Check sheet for the modelled part. Datum: model origin and axes. Units: mm. Face numbers are marked on the shaded views. A direction names the side the tool comes from. Coordinates: 2 decimals unless noted, no trailing zeros. Write each loop counter-clockwise with the first axis right and the second up, starting at its lowest first coordinate (ties: lowest second). Pieces come first, ordered by that corner, then holes. Notation, with made-up numbers: (-29, 24) - (-10, 24) arc R34 cw to (-10, 57) - close; hole circle Ø6 at (-17, 16). An arc over 180 degrees is marked (long way). Use one line per item in the form item = value. Start each with the question number.
1. Cross-section at C-C on y = 11. Record the boundary of the cut face in (x, z).
2. Cross-section at B-B on y = 5.5. Record the boundary of the cut face in (x, z), then the cut area to 3 significant figures.
3. Scan lines: line 1 along X through (y, z) = (1, -0.25); line 2 along Z through (x, y) = (-4, 1.75); line 3 along Y through (x, z) = (-2.25, 2). Record each from-to range of solid material in increasing order.
4. Go/stop test with flat-tipped pins: pin 1 Ø1 at (x, y) = (-2.5, 2.5) entering from +Z; pin 2 Ø1 at (x, z) = (-2, 2.5) entering from +Y; pin 3 Ø3 at (x, z) = (0, -3) entering from +Y. Record where each tip stops, or that it passes through.
5. Tool access check on the marked faces 4 and 5. Record the directions out of +Z, -Z, +X, -X, +Y, -Y that give a thin tool (end or side, any length) a straight path to the whole face; none if there is none.
6. Draft check along Z on the marked faces 1, 2 and 3. Enter one of: +Z half, -Z half, draft (parallel to the pull), parting line (faces both ways), or undercut.
7. Cross-section at A-A on x = -2.75. Record the boundary of the cut face in (y, z).
```python
from build123d import *

# Parameters (mm, degrees)
REVOLVE1_ANGLE          = 45
SKETCH3_W               = 5
SKETCH3_H               = 5
BOSS_EXTRUDE2_DEPTH     = 5
CHAMFER2_SIZE           = 1.5
CUT_EXTRUDE1_DEPTH      = 1
CUT_EXTRUDE1_DEPTH_BACK = 13.35


with BuildPart() as part:
    # Sketch2 → Revolve1 (revolve, symmetric)
    with BuildSketch(Plane.XY) as revolve1_sk:
        Polygon((0, 0), (5, 0), (5, 12.35), (2.5, 12.35), (2.5, 9.85), (0, 7.35), align=None)
    revolve(axis=Axis((-10, 0, 0), (0, 1, 0)), revolution_arc=REVOLVE1_ANGLE / 2)
    revolve(revolve1_sk.sketch, axis=Axis((-10, 0, 0), (0, -1, 0)), revolution_arc=REVOLVE1_ANGLE / 2)

    # Sketch3 → Boss-Extrude2 (add)
    with BuildSketch(Plane(origin=(0, 0, 0), x_dir=(0, 0, -1), z_dir=(1, 0, 0))):
        with Locations((0, 2.5)):
            Rectangle(SKETCH3_W, SKETCH3_H)
    extrude(amount=-BOSS_EXTRUDE2_DEPTH)

    # Chamfer2
    chamfer2_edges = [part.edges().sort_by_distance(p)[0] for p in [
        (-2.658770817, 0, -2.5),
        (-2.658770817, 0, 2.5),
    ]]
    chamfer(chamfer2_edges, length=CHAMFER2_SIZE)

    # Sketch4 → Cut-Extrude1 (cut, two sides)
    with BuildSketch(Plane.XZ) as cut_extrude1_sk:
        with BuildLine():
            Line((-0.761204675, 3.826834324), (4.503631926, 3.826834324))
            ThreePointArc((4.503631926, 3.826834324), (4.213147766, 4.794416604), (3.858192988, 5.740251485))
            Line((3.858192988, 5.740251485), (-0.761204675, 3.826834324))
        make_face()
        with BuildLine():
            Line((-0.761204675, -3.826834324), (4.503631926, -3.826834324))
            ThreePointArc((4.503631926, -3.826834324), (4.213147766, -4.794416604), (3.858192988, -5.740251485))
            Line((3.858192988, -5.740251485), (-0.761204675, -3.826834324))
        make_face()
    extrude(amount=CUT_EXTRUDE1_DEPTH, mode=Mode.SUBTRACT)
    extrude(cut_extrude1_sk.sketch, amount=-CUT_EXTRUDE1_DEPTH_BACK, mode=Mode.SUBTRACT)


solid = part.part
```
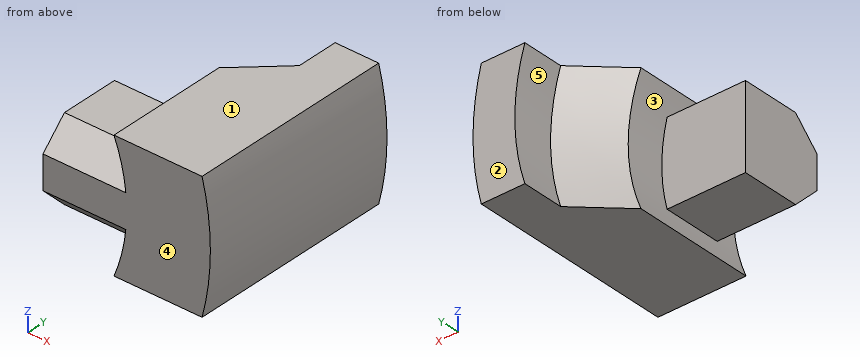
Final values:
q1.outline = (1.9, -3.83) - (4.5, -3.83) arc R15 ccw to (4.5, 3.83) - (1.9, 3.83) arc R12.5 cw to start
q2.outline = (-0.76, -3.83) - (4.5, -3.83) arc R15 ccw to (4.5, 3.83) - (-0.76, 3.83) arc R10 cw to start
q2.area = 38.9 mm²
q3.line_1 = -5 to 5
q3.line_2 = -2.5 to 2.5
q3.line_3 = 1 to 5
q4.pin_1 = 2.5
q4.pin_2 = 5
q4.pin_3 = 9.29
q5.face_4 = +Z, -Z, +X, -X, -Y
q5.face_5 = -X, +Y
q6.face_1 = +Z half
q6.face_2 = draft
q6.face_3 = undercut
q7.outline = (0, -1) - (1.5, -2.5) - (5, -2.5) - (5, 2.5) - (1.5, 2.5) - (0, 1) - close
